Geometry check sheet. Reference: drawing and pictorial views, mm from the part's lowest x, y, z. A direction names the side the tool comes from. Give positions to 0.01 mm unless a question says otherwise; leave off trailing zeros. Loops run counter-clockwise (first coordinate to the right, second up) from the corner with the lowest first, then second, coordinate; pieces in that order, holes last. Notation, with made-up numbers: (-15.75, 67) -> (38.25, 67) arc R20 cw to (38.25, 73) -> close; hole circle Ø5 at (-13.5, 52.5). An arc over 180 degrees is marked (long way). One line per item, written item: value. Start each with the question number.
(1) Sectioned sample at A-A, the plane z = 20.75. Record the cut outline in (x, y) (3 decimals), then the cut area to 3 significant figures.
(2) Sectioned sample at B-B, the plane x = 7. Record the cut outline in (y, z).
(3) Scan lines: line 1 along X through (y, z) = (30.48, 16.75); line 2 along Y through (x, z) = (8.89, 18.5); line 3 along X through (y, z) = (7, 22.5) (3 decimals). Record each from-to range of solid material in increasing order. Write a range as from..to.
(4) Sectioned sample at C-C, the plane y = 30.48. Record the cut outline in (x, z), then the cut area to 3 significant figures.
(5) Tool access check on the marked faces 4, 5 and 6. Record the directions out of +Z, -Z, +X, -X, +Y, -Y that give a thin tool (end or side, any length) a straight path to the whole face; none if there is none.
(6) Draft check along Y on the marked faces 1, 2 and 3. Enter one of: pulls with the +Y half, pulls with the -Y half, needs draft (parallel to the pull), parting line crosses it, or undercut.
(7) Sectioned sample at D-D, the plane z = 15.5. Record the cut outline in (x, y) (1 decimal), then the cut area to 3 significant figures.
(8) Gauge pin test, flat ends, axial feed: pin 1 Ø2 at (x, z) = (18.5, 15) entering from -Y; pin 2 Ø4 at (x, z) = (15, 12) entering from +Y (3 decimals). Record the tip position at first contact, or that the pin passes through.
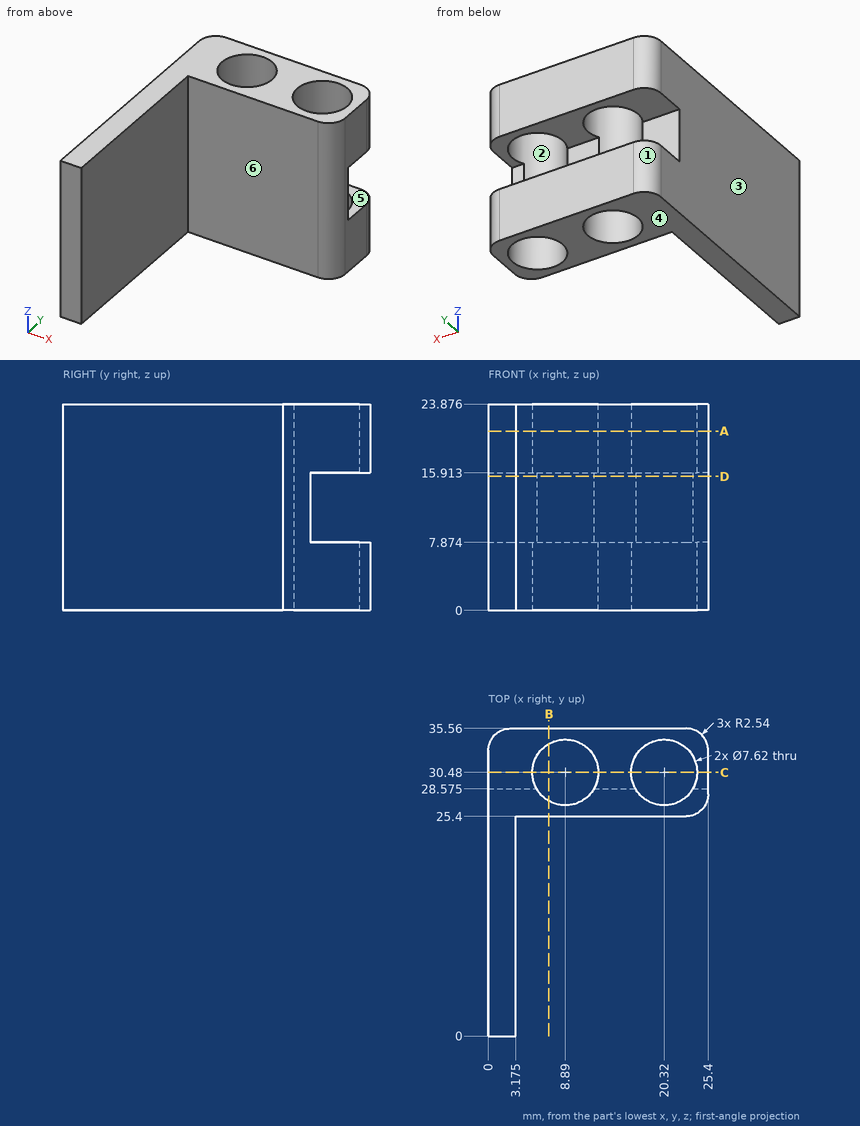
Calculated:
1. outline: (0, 0) -> (3.175, 0) -> (3.175, 25.4) -> (22.86, 25.4) arc R2.54 ccw to (25.4, 27.94) -> (25.4, 33.02) arc R2.54 ccw to (22.86, 35.56) -> (2.54, 35.56) arc R2.54 ccw to (0, 33.02) -> close; hole circle Ø7.62 at (8.89, 30.48); hole circle Ø7.62 at (20.32, 30.48)
1. area: 243 mm2
2. outline: (25.4, 0) -> (27.17, 0) -> (27.17, 23.88) -> (25.4, 23.88) -> close; (33.79, 0) -> (35.56, 0) -> (35.56, 7.87) -> (33.79, 7.87) -> close; (33.79, 15.91) -> (35.56, 15.91) -> (35.56, 23.88) -> (33.79, 23.88) -> close
3. line 1: x = 0..5.08, 12.7..16.51, 24.13..25.4
3. line 2: y = 25.4..26.67, 34.29..35.56
3. line 3: x = 0..3.175
4. outline: (0, 0) -> (5.08, 0) -> (5.08, 7.87) -> (0, 7.87) -> close; (0, 15.91) -> (5.08, 15.91) -> (5.08, 23.88) -> (0, 23.88) -> close; (12.7, 0) -> (16.51, 0) -> (16.51, 7.87) -> (12.7, 7.87) -> close; (12.7, 15.91) -> (16.51, 15.91) -> (16.51, 23.88) -> (12.7, 23.88) -> close; (24.13, 0) -> (25.4, 0) -> (25.4, 7.87) -> (24.13, 7.87) -> close; (24.13, 15.91) -> (25.4, 15.91) -> (25.4, 23.88) -> (24.13, 23.88) -> close
4. area: 161 mm2
5. face 4: -Z, +X, -X, +Y, -Y
5. face 5: +X, -X, +Y
5. face 6: +Z, -Z, +X, -Y
6. face 1: pulls with the +Y half
6. face 2: undercut
6. face 3: needs draft
7. outline: (0, 0) -> (3.2, 0) -> (3.2, 25.4) -> (22.9, 25.4) arc R2.5 ccw to (25.4, 27.9) -> (25.4, 28.6) -> (23.6, 28.6) arc R3.8 cw to (17, 28.6) -> (12.2, 28.6) arc R3.8 cw to (5.6, 28.6) -> (0, 28.6) -> close
7. area: 142 mm2
8. pin 1: stops at y = 25.4
8. pin 2: stops at y = 28.575
